from build123d import *

# Parameters (mm, degrees)
BOSS_EXTRUDE1_DEPTH          = 50.8
SKETCH2_R                    = 3.4
M8X1_25_THREADED_HOLES_DEPTH = 50.8
CUT_EXTRUDE2_REACH           = 75.634
SKETCH3_R                    = 3.2639


with BuildPart() as part:
    # Sketch1 → Boss-Extrude1 (new body)
    with BuildSketch(Plane.XY):
        Polygon((0, 1.791647537), (0, 34.811647537), (41.845257966, 34.811647537), (41.845257966, 28.3636723), (9.525, 28.3636723), (9.525, 7.7134723), (41.845257966, 7.7134723), (41.845257966, 1.791647537), align=None)
    extrude(amount=BOSS_EXTRUDE1_DEPTH)

    # Sketch2 → M8x1.25 Threaded Holes (cut)
    with BuildSketch(Plane(origin=(9.525, 0, 0), x_dir=(0, 0, -1), z_dir=(1, 0, 0))):
        with Locations((-38.1, 21.430460881)):
            Circle(SKETCH2_R)
        with Locations((-12.7, 21.430460881)):
            Circle(SKETCH2_R)
    extrude(amount=-M8X1_25_THREADED_HOLES_DEPTH, mode=Mode.SUBTRACT)

    # Cut-Extrude2: up to this face of the body (flat: up to its plane)
    cut_extrude2_end = Plane(part.part.faces().sort_by_distance((20.922628983, 1.791647537, 25.4))[0])
    # Sketch3 → Cut-Extrude2 (cut, up to the picked face)
    with BuildSketch(Plane(origin=(0, 34.811647537, 0), x_dir=(1, 0, 0), z_dir=(0, 1, 0)), mode=Mode.PRIVATE) as cut_extrude2_sk1:
        with Locations(Location((29.145257966, -25.4, 0), (0, 0, 270))):
            Circle(SKETCH3_R)
    cut_extrude2_tool1 = split(extrude(cut_extrude2_sk1.sketch, amount=-CUT_EXTRUDE2_REACH, mode=Mode.PRIVATE), bisect_by=cut_extrude2_end, keep=Keep.BOTH, mode=Mode.PRIVATE)
    # Sketch3 → Cut-Extrude2 (cut, up to the picked face)
    with BuildSketch(Plane(origin=(0, 34.811647537, 0), x_dir=(1, 0, 0), z_dir=(0, 1, 0)), mode=Mode.PRIVATE) as cut_extrude2_sk2:
        Polygon((12.7, 0), (37.489157966, -17.78), (37.489157966, -33.02), (12.7, -50.8), (41.845257966, -50.8), (41.845257966, 0), align=None)
    cut_extrude2_tool2 = split(extrude(cut_extrude2_sk2.sketch, amount=-CUT_EXTRUDE2_REACH, mode=Mode.PRIVATE), bisect_by=cut_extrude2_end, keep=Keep.BOTH, mode=Mode.PRIVATE)
    add(cut_extrude2_tool1.solids().sort_by(Axis((29.145258, 34.811648, 25.4), (0, -1, 0)))[0], mode=Mode.SUBTRACT)
    add(cut_extrude2_tool2.solids().sort_by(Axis((25.435926, 34.811648, 8.414089), (0, -1, 0)))[0], mode=Mode.SUBTRACT)


solid = part.part
Model file for the job. Use its own axes, mm. A direction names the side the tool comes from. Coordinates: 2 decimals unless noted, no trailing zeros. Write each loop counter-clockwise with the first axis right and the second up, starting at its lowest first coordinate (ties: lowest second). Pieces come first, ordered by that corner, then holes. Notation, with made-up numbers: (-19.75, -15) -> (-1.75, -15) arc R24 ccw to (-1.75, 18) -> close; hole circle Ø9 at (69, -20.75). An arc over 180 degrees is marked (long way). One line per item, written item: value. Start each with the question number.
1) Slice it at C-C on z = 15. Write the cut outline in (x, y) (3 decimals), then the cut area to 3 significant figures.
2) Probe probe 1 along Y at (x, z) = (32.5, 34); probe 2 along X at (y, z) = (6.35, 25.4); probe 3 along Z at (x, y) = (7, 19). List the from-to ranges inside material, lowest first.
3) Pull direction Y, two halves, no side cores. Call faces 1 (the face through (21, 28.364, 25)), 2 (the face through (37.489, 32, 25)), 3 (the face through (15, 1.792, 25)): +Y half, -Y half, draft (parallel to the pull), parting line (faces both ways), or undercut.
4) Which spindle directions (+Z, -Z, +X, -X, +Y, -Y) get a long thin tool onto all of the face, cutting with end or side? Do faces 4 (the face through (9.525, 18, 25)), 5 (the face through (37.489, 5, 25)). Say none if no direction does.
5) Slice it at D-D on y = 30. Write the cut outline in (x, z), then the cut area to 3 significant figures.
6) Slice it at B-B on x = 31.5. Write the cut outline in (y, z).
7) Flat gauge pins, fed straight in: pin 1 Ø5.5 at (y, z) = (21.43, 38.1) entering from +X; pin 2 Ø6 at (y, z) = (14.5, 28) entering from +X (3 decimals). Where does each tip first touch, or does it go through?
8) Slice it at A-A on z = 25.4. Write the cut outline in (x, y) (3 decimals).
Answers follow:
1. outline: (0, 1.792) -> (33.613, 1.792) -> (33.613, 7.713) -> (9.525, 7.713) -> (9.525, 18.926) -> (0, 18.926) -> close; (0, 23.934) -> (9.525, 23.934) -> (9.525, 28.364) -> (33.613, 28.364) -> (33.613, 34.812) -> (0, 34.812) -> close
1. area: 565 mm2
2. probe 1: 1.79 to 7.71, 28.36 to 34.81
2. probe 2: 0 to 25.88, 32.41 to 37.49
2. probe 3: 0 to 10.32, 15.08 to 35.72, 40.48 to 50.8
3. face 1: undercut
3. face 2: draft
3. face 3: -Y half
4. face 4: +Z, -Z, +X
4. face 5: +Z, -Z, +X, +Y, -Y
5. outline: (0, 0) -> (12.7, 0) -> (37.49, 17.78) -> (37.49, 33.02) -> (12.7, 50.8) -> (0, 50.8) -> close; hole circle Ø6.53 at (29.15, 25.4)
5. area: 1,430 mm2
6. outline: (1.79, 13.48) -> (7.71, 13.48) -> (7.71, 23.14) -> (1.79, 23.14) -> close; (1.79, 27.66) -> (7.71, 27.66) -> (7.71, 37.32) -> (1.79, 37.32) -> close; (28.36, 13.48) -> (34.81, 13.48) -> (34.81, 23.14) -> (28.36, 23.14) -> close; (28.36, 27.66) -> (34.81, 27.66) -> (34.81, 37.32) -> (28.36, 37.32) -> close
7. pin 1: through
7. pin 2: x = 9.525
8. outline: (0, 1.792) -> (25.881, 1.792) -> (25.881, 7.713) -> (9.525, 7.713) -> (9.525, 28.364) -> (25.881, 28.364) -> (25.881, 34.812) -> (0, 34.812) -> close; (32.409, 1.792) -> (37.489, 1.792) -> (37.489, 7.713) -> (32.409, 7.713) -> close; (32.409, 28.364) -> (37.489, 28.364) -> (37.489, 34.812) -> (32.409, 34.812) -> close
